Verification items for the finished model (mm, model axes). A direction names the side the tool comes from. Coordinates: 2 decimals unless noted, no trailing zeros. Order: outer loops, then holes, each group sorted by start corner. A loop starts at its lowest first (then second) coordinate and runs counter-clockwise, first axis right, second up. Notation, with made-up numbers: (69.5, -13.75) -> (89.5, -13.75) arc R24 cw to (89.5, -1.75) -> close; hole circle Ø2 at (67.25, -38). An arc over 180 degrees is marked (long way). Use CSV: the item, a comma, the result in double quotes. Start each with the question number.
1) Sectioned sample at B-B on x = -20. Record the boundary of the cut face in (y, z).
2) Release check for a two-part mould opening along Y. For faces 4 (the flat face through (-21, -49.514, 6)), 5 (the flat face through (-20, 65, 3)), 6 (the flat face through (-21, 14, 0)), 7 (the cylindrical face through (-20.08, 75.74, 5.92)) record: released by +Y, released by -Y, zero draft, split by the parting line, or undercut.
3) Scan lines: line 1 along Y through (x, z) = (-20.5, 9.5); line 2 along X through (y, z) = (27.5, 5); line 3 along Y through (x, z) = (-21, 8). Record each from-to range of solid material in increasing order.
4) Tool access check on faces 1 (the flat face through (-12.914, 4, 6)), 2 (the flat face through (-20, 67.986, 8)), 3 (the flat face through (-27.914, 4, 6)). Record the directions out of +Z, -Z, +X, -X, +Y, -Y that give a thin tool (end or side, any length) a straight path to the whole face; none if there is none.
5) Sectioned sample at A-A on z = 10.25. Record the boundary of the cut face in (x, y).
6) Sectioned sample at C-C on y = 38.5. Record the boundary of the cut face in (x, z).
7) Sectioned sample at D-D on x = -11.75. Record the boundary of the cut face in (y, z), then the cut area to 3 significant figures.
8) Go/stop test with flat-tipped pins: pin 1 (1.5 mm diameter, centred on y = 37, z = 2.5, fed in from -X); pin 2 (4 mm diameter, centred on x = -26.5, z = 7, fed in from +Y). Record where each tip stops, or that it passes through.
from build123d import *

# Parameters (mm, degrees)
SKETCH1_R           = 10.259142264
SKETCH1_W           = 15
SKETCH1_H           = 108
BOSS_EXTRUDE1_DEPTH = 12
SKETCH2_R           = 3.25
CUT_EXTRUDE1_DEPTH  = 9
BOSS_EXTRUDE2_DEPTH = 9


with BuildPart() as part:
    # Sketch1 → Boss-Extrude1 (new body)
    with BuildSketch(Plane.XY):
        with Locations((-20.413846154, 65.486153846)):
            Circle(SKETCH1_R)
        with Locations((-20.413846154, 4.486153846)):
            Rectangle(SKETCH1_W, SKETCH1_H)
    extrude(amount=BOSS_EXTRUDE1_DEPTH)

    # Sketch2 → Cut-Extrude1 (cut)
    with BuildSketch(Plane.XY.offset(12)):
        with Locations((-20.413846154, 65.486153846)):
            Circle(SKETCH2_R)
    extrude(amount=-CUT_EXTRUDE1_DEPTH, mode=Mode.SUBTRACT)

    # Sketch3 → Boss-Extrude2 (add)
    with BuildSketch(Plane.XY.offset(12)):
        with BuildLine():
            Line((-22.49050212, 67.986153846), (-18.337190188, 67.986153846))
            ThreePointArc((-18.337190188, 67.986153846), (-20.413846154, 68.736153846), (-22.49050212, 67.986153846))
        make_face()
    extrude(amount=-BOSS_EXTRUDE2_DEPTH)


solid = part.part
Answers follow:
1,outline,"(-49.51, 0) -> (75.74, 0) -> (75.74, 12) -> (67.99, 12) -> (67.99, 3) -> (62.26, 3) -> (62.26, 12) -> (-49.51, 12) -> close"
2,face 4,"released by -Y"
2,face 5,"undercut"
2,face 6,"zero draft"
2,face 7,"split by the parting line"
3,line 1,"y = -49.51 to 62.24, 67.99 to 75.74"
3,line 2,"x = -27.91 to -12.91"
3,line 3,"y = -49.51 to 62.29, 67.99 to 75.73"
4,face 1,"+Z, -Z, +X, -Y"
4,face 2,"+Z"
4,face 3,"+Z, -Z, -X, -Y"
5,outline,"(-27.91, -49.51) -> (-12.91, -49.51) -> (-12.91, 58.49) arc R10.26 ccw (long way) to (-27.91, 58.49) -> close; hole (-22.49, 67.99) arc R3.25 ccw (long way) to (-18.34, 67.99) -> close"
6,outline,"(-27.91, 0) -> (-12.91, 0) -> (-12.91, 12) -> (-27.91, 12) -> close"
7,outline,"(59.99, 0) -> (70.98, 0) -> (70.98, 12) -> (59.99, 12) -> close"
7,area,"132 mm²"
8,pin 1,"stops at x = -27.91"
8,pin 2,"stops at y = 74.9"
